```python
from build123d import *

# Parameters (mm, degrees)
F0_R     = 5
F0_R_2   = 2
F0_R_3   = 6.5
F0_R_4   = 2.5
F1_DEPTH = 9
F0_R_5   = 3.5
F2_DEPTH = 5


with BuildPart() as f1:
    # F0 (on Front) → F1 (new body)
    with BuildSketch(Plane.XZ):
        with BuildLine():
            Line((40, 150), (-40, 150))
            ThreePointArc((-40, 150), (-47.071068, 147.071068), (-50, 140))
            Line((-50, 140), (-50, 10))
            ThreePointArc((-50, 10), (-47.071068, 2.928932), (-40, 0))
            Line((-40, 0), (-12.5, 0))
            Line((-12.5, 0), (-12.5, 50))
            Line((-12.5, 50), (0, 50))
            Line((0, 50), (12.5, 50))
            Line((12.5, 50), (12.5, 0))
            Line((12.5, 0), (40, 0))
            ThreePointArc((40, 0), (47.071068, 2.928932), (50, 10))
            Line((50, 10), (50, 140))
            ThreePointArc((50, 140), (47.071068, 147.071068), (40, 150))
        make_face()
        with BuildLine():
            ThreePointArc((-27, 10), (-30, 7), (-33, 10))
            Line((-33, 10), (-33, 35))
            ThreePointArc((-33, 35), (-30, 38), (-27, 35))
            Line((-27, 35), (-27, 10))
        make_face(mode=Mode.SUBTRACT)
        with Locations((-40, 60)):
            Circle(F0_R, mode=Mode.SUBTRACT)
        with BuildLine():
            Line((-33, 45), (-33, 70))
            ThreePointArc((-33, 70), (-30, 73), (-27, 70))
            Line((-27, 70), (-27, 45))
            ThreePointArc((-27, 45), (-30, 42), (-33, 45))
        make_face(mode=Mode.SUBTRACT)
        with Locations((-19, 55)):
            Circle(F0_R_2, mode=Mode.SUBTRACT)
        with BuildLine():
            Line((27, 10), (27, 35))
            ThreePointArc((27, 35), (30, 38), (33, 35))
            Line((33, 35), (33, 10))
            ThreePointArc((33, 10), (30, 7), (27, 10))
        make_face(mode=Mode.SUBTRACT)
        with Locations((0, 55)):
            Circle(F0_R_2, mode=Mode.SUBTRACT)
        with Locations((19, 55)):
            Circle(F0_R_2, mode=Mode.SUBTRACT)
        with BuildLine():
            ThreePointArc((27, 70), (30, 73), (33, 70))
            Line((33, 70), (33, 45))
            ThreePointArc((33, 45), (30, 42), (27, 45))
            Line((27, 45), (27, 70))
        make_face(mode=Mode.SUBTRACT)
        with Locations((40, 60)):
            Circle(F0_R_3, mode=Mode.SUBTRACT)
        with BuildLine():
            ThreePointArc((-27, 80), (-30, 77), (-33, 80))
            Line((-33, 80), (-33, 105))
            ThreePointArc((-33, 105), (-30, 108), (-27, 105))
            Line((-27, 105), (-27, 80))
        make_face(mode=Mode.SUBTRACT)
        with Locations((-40, 137.5)):
            Circle(F0_R, mode=Mode.SUBTRACT)
        with Locations((-10, 120)):
            Circle(F0_R_4, mode=Mode.SUBTRACT)
        with Locations((-19, 145)):
            Circle(F0_R_2, mode=Mode.SUBTRACT)
        with BuildLine():
            Line((33, 105), (33, 80))
            ThreePointArc((33, 80), (30, 77), (27, 80))
            Line((27, 80), (27, 105))
            ThreePointArc((27, 105), (30, 108), (33, 105))
        make_face(mode=Mode.SUBTRACT)
        with Locations((10, 120)):
            Circle(F0_R_4, mode=Mode.SUBTRACT)
        with Locations((0, 145)):
            Circle(F0_R_2, mode=Mode.SUBTRACT)
        with Locations((19, 145)):
            Circle(F0_R_2, mode=Mode.SUBTRACT)
        with Locations((40, 137.5)):
            Circle(F0_R_3, mode=Mode.SUBTRACT)
    extrude(amount=F1_DEPTH)

    # F0 (on Front) → F2 (join)
    with BuildSketch(Plane.XZ):
        with Locations((-40, 137.5)):
            Circle(F0_R)
        with Locations((-40, 137.5)):
            Circle(F0_R_4, mode=Mode.SUBTRACT)
        with Locations((40, 137.5)):
            Circle(F0_R_3)
        with Locations((40, 137.5)):
            Circle(F0_R_5, mode=Mode.SUBTRACT)
        with Locations((40, 60)):
            Circle(F0_R_3)
        with Locations((40, 60)):
            Circle(F0_R_5, mode=Mode.SUBTRACT)
        with Locations((-40, 60)):
            Circle(F0_R)
        with Locations((-40, 60)):
            Circle(F0_R_4, mode=Mode.SUBTRACT)
    extrude(amount=F2_DEPTH)


solid = f1.part
```
Design review of the part built by this model. Coordinates are the model's own, in mm. A direction names the side the tool comes from. Give positions to 0.01 mm unless a question says otherwise; leave off trailing zeros. Order: outer loops, then holes, each group sorted by start corner. A loop starts at its lowest first (then second) coordinate and runs counter-clockwise, first axis right, second up. Notation, with made-up numbers: M 65.5,-12 L 90.5,-12 A9 ccw 90.5,4 Z; hole C 84,-23 d6. An arc over 180 degrees is marked long. One line per question, with ' | ' between items. Start each with the question number.
Q1. For L1, parallel to X at y = -7.75, z = 138; L2, parallel to X at y = -4.5, z = 95.5; L3, parallel to Z at x = 40, y = -4.75, list the stretches that pass through material, from the lowest coordinate up. Write a range as [from, to].
Q2. For pin 1 Ø3 at (x, z) = (19, 55) entering from -Y; pin 2 Ø6.5 at (x, z) = (41, 59) entering from -Y; pin 3 Ø2.5 at (x, y) = (-5, -6) entering from -Z, all flat-tipped, find the tip position at first contact; note any pin that passes through.
Q3. We need section D-D (x = 30). Write out the cut boundary in (y, z).
Q4. We need section B-B (x = -19). Write out the cut boundary in (y, z), plus the area to 3 significant figures.
Q5. We need section C-C (z = 60). Write out the cut boundary in (x, y).
Q6. We need section A-A (z = 137.5). Write out the cut boundary in (x, y).
Q7. The part is to be moulded in two halves that separate along X. For faces 6 (the face through (50, -4, 74)), 7 (the face through (26, -4, 0)), 8 (the face through (30, -4, 108)), say which applies: +X half, -X half, draft (parallel to the pull), parting line (faces both ways), or undercut.
Q8. Machinability: for faces 1 (the face through (38.591, -6.972, 53.655)), 2 (the face through (12.5, -4, 25)), 3 (the face through (-50, -4, 76)), 4 (the face through (-1, -9, 76)), 5 (the face through (30, -4, 77)), which of the approach directions +Z, -Z, +X, -X, +Y, -Y give a long, thin tool a straight path to every point of the face, cutting with its end or side? Answer none if there is none.
Returned:
1) L1: [-50, -44.97], [-35.03, 33.52], [46.48, 50] | L2: [-50, -33], [-27, 27], [33, 50] | L3: [0, 56.5], [63.5, 134], [141, 150]
2) pin 1: through | pin 2: y = -5 | pin 3: z = 50
3) outline: M -9,0 L 0,0 L 0,7 L -9,7 Z; M -9,38 L 0,38 L 0,42 L -9,42 Z; M -9,73 L 0,73 L 0,77 L -9,77 Z; M -9,108 L 0,108 L 0,150 L -9,150 Z
4) outline: M -9,0 L 0,0 L 0,53 L -9,53 Z; M -9,57 L 0,57 L 0,143 L -9,143 Z; M -9,147 L 0,147 L 0,150 L -9,150 Z | area: 1,280 mm2
5) outline: M -50,-9 L -45,-9 L -45,-5 L -42.5,-5 L -42.5,0 L -50,0 Z; M -37.5,-5 L -35,-5 L -35,-9 L -33,-9 L -33,0 L -37.5,0 Z; M -27,-9 L 27,-9 L 27,0 L -27,0 Z; M 33,-9 L 33.5,-9 L 33.5,-5 L 36.5,-5 L 36.5,0 L 33,0 Z; M 43.5,-5 L 46.5,-5 L 46.5,-9 L 50,-9 L 50,0 L 43.5,0 Z
6) outline: M -50,-9 L -45,-9 L -45,-5 L -42.5,-5 L -42.5,0 L -50,0 Z; M -37.5,-5 L -35,-5 L -35,-9 L 33.5,-9 L 33.5,-5 L 36.5,-5 L 36.5,0 L -37.5,0 Z; M 43.5,-5 L 46.5,-5 L 46.5,-9 L 50,-9 L 50,0 L 43.5,0 Z
7) face 6: +X half | face 7: draft | face 8: undercut
8) face 1: -Y | face 2: -Z, +Y, -Y | face 3: +Z, -Z, -X, +Y, -Y | face 4: +Z, -Z, +X, -X, -Y | face 5: +Y, -Y
